from build123d import *

# Parameters (mm, degrees)
SKETCH009_W     = 31
SKETCH009_H     = 31.5
PAD001_DEPTH    = 21
SKETCH010_W     = 18
SKETCH010_H     = 6
POCKET007_DEPTH = 19.4
PAD002_DEPTH    = 3.65
SKETCH012_W     = 9
SKETCH012_H     = 9
POCKET008_DEPTH = 2.15


with BuildPart() as part:
    # Sketch009 → Pad001 (new body)
    with BuildSketch(Plane.XY):
        with Locations((0, 9.25)):
            Rectangle(SKETCH009_W, SKETCH009_H)
    extrude(amount=PAD001_DEPTH)

    # Sketch010 → Pocket007 (cut)
    with BuildSketch(Plane.XY):
        Polygon((-7.9, -2.85), (-7.9, -1), (-10.5, -1), (-10.5, -2.85), (-13.2, -2.85), (-13.2, -0.65), (-13.7, -0.65), (-13.7, 0.65), (-13.2, 0.65), (-13.2, 23.45), (13.2, 23.45), (13.2, 0.65), (13.7, 0.65), (13.7, -0.65), (13.2, -0.65), (13.2, -2.85), (10.5, -2.85), (10.5, -1), (7.9, -1), (7.9, -2.85), align=None)
        with Locations((0, 7.45)):
            Rectangle(SKETCH010_W, SKETCH010_H, mode=Mode.SUBTRACT)
    extrude(amount=POCKET007_DEPTH, mode=Mode.SUBTRACT)

    # Sketch011 → Pad002 (join)
    with BuildSketch(Plane.XZ.offset(2.85)):
        with BuildLine():
            Line((-7.75, 0), (-5.05, -11.85))
            Line((-5.05, -11.85), (-4, -11.85))
            ThreePointArc((4, -11.85), (0, -7.85), (-4, -11.85))
            Line((4, -11.85), (5.05, -11.85))
            Line((5.05, -11.85), (7.75, 0))
            Line((7.75, 0), (-7.75, 0))
        make_face()
    extrude(amount=PAD002_DEPTH)

    # Sketch012 → Pocket008 (cut)
    with BuildSketch(Plane.XZ.offset(2.85)):
        with Locations((0, -12)):
            Rectangle(SKETCH012_W, SKETCH012_H)
    extrude(amount=POCKET008_DEPTH, mode=Mode.SUBTRACT)


with BuildPart() as part_1:
    # Body001 placement: moved
    add(part.part.moved(Location((0, 0, 12))))


solid = part_1.part
Work out the finished part from the listing and answer in its coordinate system (mm). A direction names the side the tool comes from. Give positions to 0.01 mm unless a question says otherwise; leave off trailing zeros. Order: outer loops, then holes, each group sorted by start corner. A loop starts at its lowest first (then second) coordinate and runs counter-clockwise, first axis right, second up. Notation, with made-up numbers: (40, 11.5) -> (61, 11.5) arc R8 ccw to (61, 15.5) -> close; hole circle Ø3 at (22.5, 27.25). An arc over 180 degrees is marked (long way). Answer as a JSON object with one key per item and string values. Group by question number.
1. Section D-D on y = 8.5 is taken. Determine the outline of the cut face in (x, z).
2. Consider line 1 along Y through (x, z) = (-5, 22); line 2 along X through (y, z) = (-1.5, 26); line 3 along X through (y, z) = (9, 18.5). Determine where each line is inside the solid, lowest interval first. Write a range as [from, to].
3. The mould has two halves that part along Y. Classify faces 1 (the flat face through (12, -2.85, 22)), 2 (the flat face through (0, 25, 22)), 3 (the flat face through (-6.42, -4.65, 6.16)): released by +Y, released by -Y, zero draft, split by the parting line, or undercut.
4. Section C-C on x = 0 is taken. Determine the outline of the cut face in (y, z).
5. Flat-ended cylindrical pins translate along their axes: pin 1 Ø1.5 at (x, y) = (-1, 6.5) entering from -Z; pin 2 Ø4 at (x, y) = (6.5, 16) entering from -Z. Find the tip coordinate at first contact, or state that the pin passes through.
6. A tool of negligible diameter and unlimited length cuts with its end or side. For faces 4 (the flat face through (-7.9, -2, 22)), 5 (the flat face through (0, 7, 12)), 6 (the flat face through (4.5, -4, 2)), 7 (the flat face through (6.38, -4.65, 5.99)), from which of +Z, -Z, +X, -X, +Y, -Y can it reach the whole face along a straight path? Write none if from no direction.
7. Section B-B on y = 0 is taken. Determine the outline of the cut face in (x, z), plus the area to 3 significant figures.
8. Section A-A on z = 21 is taken. Determine the outline of the cut face in (x, y).
Result sheet:
{
 "1": {"outline": "(-15.5, 12) -> (-13.2, 12) -> (-13.2, 31.4) -> (-9, 31.4) -> (-9, 12) -> (9, 12) -> (9, 31.4) -> (13.2, 31.4) -> (13.2, 12) -> (15.5, 12) -> (15.5, 33) -> (-15.5, 33) -> close"},
 "2": {"line 1": "y = [-6.5, -2.85], [4.45, 10.45], [23.45, 25]", "line 2": "x = [-15.5, -13.2], [-10.5, -7.9], [7.9, 10.5], [13.2, 15.5]", "line 3": "x = [-15.5, -13.2], [-9, 9], [13.2, 15.5]"},
 "3": {"face 1": "undercut", "face 2": "released by +Y", "face 3": "zero draft"},
 "4": {"outline": "(-6.5, 4.15) -> (-5, 4.15) -> (-5, 4.5) -> (-2.85, 4.5) -> (-2.85, 31.4) -> (4.45, 31.4) -> (4.45, 12) -> (10.45, 12) -> (10.45, 31.4) -> (23.45, 31.4) -> (23.45, 12) -> (25, 12) -> (25, 33) -> (-6.5, 33) -> close"},
 "5": {"pin 1": "stops at z = 12", "pin 2": "stops at z = 31.4"},
 "6": {"face 4": "-Z", "face 5": "-Z, +X, -X, +Y", "face 6": "-Z, +Y", "face 7": "-Z, +X, +Y, -Y"},
 "7": {"outline": "(-15.5, 12) -> (-13.7, 12) -> (-13.7, 31.4) -> (13.7, 31.4) -> (13.7, 12) -> (15.5, 12) -> (15.5, 33) -> (-15.5, 33) -> close", "area": "119 mm^2"},
 "8": {"outline": "(-15.5, -6.5) -> (15.5, -6.5) -> (15.5, 25) -> (-15.5, 25) -> close; (-9, 4.45) -> (9, 4.45) -> (9, 10.45) -> (-9, 10.45) -> close; hole (-13.7, -0.65) -> (-13.2, -0.65) -> (-13.2, -2.85) -> (-10.5, -2.85) -> (-10.5, -1) -> (-7.9, -1) -> (-7.9, -2.85) -> (7.9, -2.85) -> (7.9, -1) -> (10.5, -1) -> (10.5, -2.85) -> (13.2, -2.85) -> (13.2, -0.65) -> (13.7, -0.65) -> (13.7, 0.65) -> (13.2, 0.65) -> (13.2, 23.45) -> (-13.2, 23.45) -> (-13.2, 0.65) -> (-13.7, 0.65) -> close"}
}
